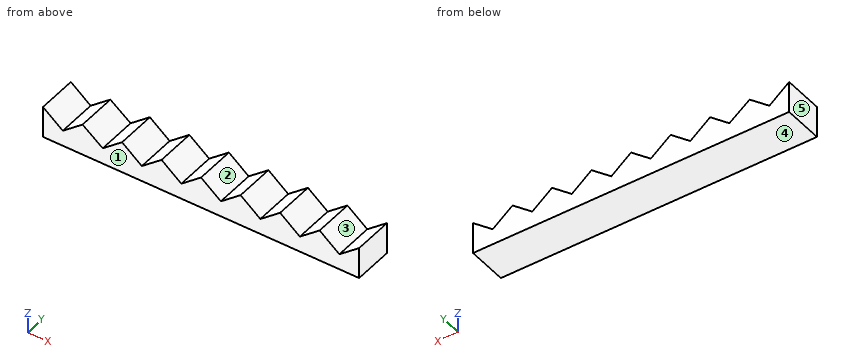
```python
from build123d import *

# Parameters (mm, degrees)
F1_DEPTH = 6.35
F2_SCALE = 2


with BuildPart() as f1:
    # F0 (on Front) → F1 (new body)
    with BuildSketch(Plane.XZ):
        Polygon((19.05, -2.54), (25.4, -2.54), (25.4, 2.54), (22.225, 0), (19.05, 2.54), (15.875, 0), (12.7, 2.54), (9.525, 0), (6.35, 2.54), (3.175, 0), (0, 2.54), (-3.175, 0), (-6.35, 2.54), (-9.525, 0), (-12.7, 2.54), (-15.8026084123, 0.0579132702), (-19.05, 2.54), (-22.225, 0), (-25.4, 2.54), (-25.4, -2.54), (-19.05, -2.54), (-12.7, -2.54), (-6.35, -2.54), (0, -2.54), (6.35, -2.54), (12.7, -2.54), align=None)
    extrude(amount=F1_DEPTH)


with BuildPart() as f1_1:
    # F2: moved
    add(f1.part.scale(F2_SCALE))


solid = f1_1.part
```
The model under review builds one solid part; all positions refer to its coordinate system, in mm. Face numbers are marked on the shaded views. A direction names the side the tool comes from. Give positions to 0.01 mm unless a question says otherwise; leave off trailing zeros. Write each loop counter-clockwise with the first axis right and the second up, starting at its lowest first coordinate (ties: lowest second). Pieces come first, ordered by that corner, then holes. Notation, with made-up numbers: (44.5, -18.5) -> (50.5, -18.5) arc R8 ccw to (50.5, -12.5) -> close; hole circle Ø9 at (1, -26). An arc over 180 degrees is marked (long way). Answer in a Markdown table with one row per item.
1) Add section C-C on x = 14. State the section outline as (y, z) points, plus the area to 3 significant figures.
Worked answers:
| item | result |
|---|---|
| outline | (-12.7, -5.08) -> (0, -5.08) -> (0, 4.04) -> (-12.7, 4.04) -> close |
| area | 116 mm² |
2) Tool access review of the marked faces 1 and 2: name each direction out of +Z, -Z, +X, -X, +Y, -Y from which nothing blocks a thin tool from reaching the whole face with its end or side.
Worked answers:
| item | result |
|---|---|
| face 1 | +Z, -Z, +X, -X, -Y |
| face 2 | +Z, +Y, -Y |
3) Clearance check with a flat-ended pin moving along its axis: P1, Ø3, axis at x = 4, y = -10.5, coming from the +Z side. State where the tip first meets the part, or that it passes through.
Worked answers:
| item | result |
|---|---|
| P1 | z = 3.08 |
4) Add section D-D on x = -5. State the section outline as (y, z) points, plus the area to 3 significant figures.
Worked answers:
| item | result |
|---|---|
| outline | (-12.7, -5.08) -> (0, -5.08) -> (0, 1.08) -> (-12.7, 1.08) -> close |
| area | 78.2 mm² |
5) For L1, parallel to Z at x = -43, y = -9; L2, parallel to Z at x = 47, y = -6, list the stretches that pass through material, from the lowest coordinate up. Write a range as [from, to].
Worked answers:
| item | result |
|---|---|
| L1 | [-5.08, 1.16] |
| L2 | [-5.08, 2.04] |
6) Add section B-B on z = 2.25. Count the separate pieces of the cut face and the enclosed holes in it, plus the area to 3 significant figures.
Worked answers:
| item | result |
|---|---|
| separate pieces | 9 |
| enclosed holes | 0 |
| area | 721 mm² |
7) Add section A-A on y = -10.75. State the section outline as (x, z) points, plus the area to 3 significant figures.
Worked answers:
| item | result |
|---|---|
| outline | (-50.8, -5.08) -> (50.8, -5.08) -> (50.8, 5.08) -> (44.45, 0) -> (38.1, 5.08) -> (31.75, 0) -> (25.4, 5.08) -> (19.05, 0) -> (12.7, 5.08) -> (6.35, 0) -> (0, 5.08) -> (-6.35, 0) -> (-12.7, 5.08) -> (-19.05, 0) -> (-25.4, 5.08) -> (-31.61, 0.12) -> (-38.1, 5.08) -> (-44.45, 0) -> (-50.8, 5.08) -> close |
| area | 775 mm² |
8) Mouldability with a two-part tool opening along X and no side actions: class the marked faces 3, 4 and 5 as +X half, -X half, draft (parallel to the pull), parting line (faces both ways), or undercut.
Worked answers:
| item | result |
|---|---|
| face 3 | undercut |
| face 4 | draft |
| face 5 | -X half |
